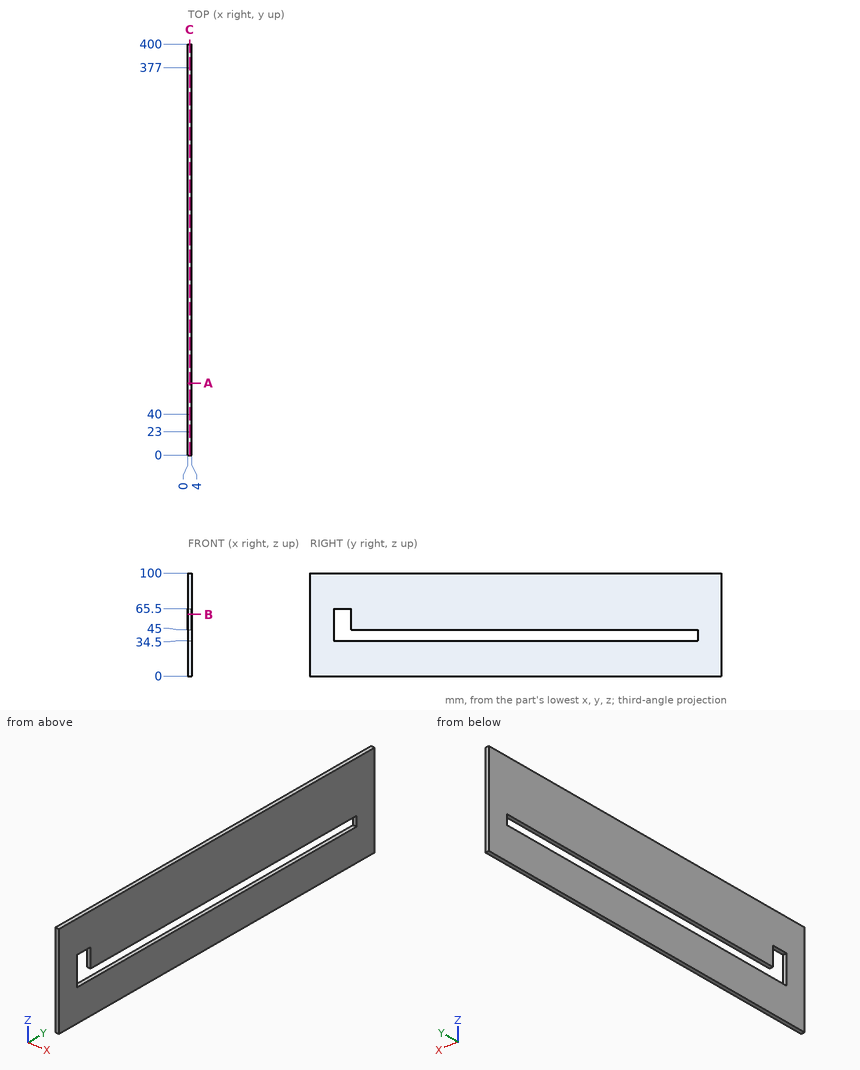
Job drawing, mm, ordinate dimensions from the low corner. One solid piece. Round coordinates to 2 decimals unless told otherwise and drop trailing zeros. Write each loop counter-clockwise with the first axis right and the second up, starting at its lowest first coordinate (ties: lowest second). Pieces come first, ordered by that corner, then holes. Notation, with made-up numbers: (63, 25.25) -> (95, 25.25) arc R24 ccw to (95, 38.25) -> close; hole circle Ø9 at (49.25, 27.5). An arc over 180 degrees is marked (long way). Answer as a JSON object with one key per item and string values.
(1) Band-saw the part on C-C, the plane x = 1.75. List the corners of the cut face in (y, z), then the cut area to 3 significant figures.
Reported:
{"outline": "(0, 0) -> (400, 0) -> (400, 100) -> (0, 100) -> close; hole (23, 34.5) -> (377, 34.5) -> (377, 45) -> (40, 45) -> (40, 65.5) -> (23, 65.5) -> close", "area": "35,900 mm^2"}
(2) Band-saw the part on B-B, the plane z = 60. List the corners of the cut face in (x, y), then the cut area to 3 significant figures.
Reported:
{"outline": "(0, 0) -> (4, 0) -> (4, 23) -> (0, 23) -> close; (0, 40) -> (4, 40) -> (4, 400) -> (0, 400) -> close", "area": "1,530 mm^2"}
(3) Band-saw the part on A-A, the plane y = 70. List the corners of the cut face in (x, z).
Reported:
{"outline": "(0, 0) -> (4, 0) -> (4, 34.5) -> (0, 34.5) -> close; (0, 45) -> (4, 45) -> (4, 100) -> (0, 100) -> close"}
(4) Pin check, flat tip, straight feed: P1, Ø5, axis at y = 204.5, z = 29.5, coming from the -X side. Stop position of the tip, or through.
Reported:
{"P1": "stops at x = 0"}
(5) Probe probe 1 along Z at (x, y) = (3.75, 179.5); probe 2 along Y at (x, z) = (3, 53.5); probe 3 along Y at (x, z) = (0.4, 39.5). List the from-to ranges inside material, lowest first. Write a range as [from, to].
Reported:
{"probe 1": "z = [0, 34.5], [45, 100]", "probe 2": "y = [0, 23], [40, 400]", "probe 3": "y = [0, 23], [377, 400]"}
